from build123d import *

# Parameters (mm, degrees)
BOSS_EXTRUDE1_DEPTH = 60
CUT_EXTRUDE1_DEPTH  = 41
SKETCH3_W           = 20
SKETCH3_H           = 20
CUT_EXTRUDE2_DEPTH  = 10
CHAMFER1_SIZE       = 20
SKETCH4_W           = 10
SKETCH4_H           = 20
CUT_EXTRUDE3_DEPTH  = 30
SKETCH5_W           = 10
SKETCH5_H           = 20
CUT_EXTRUDE4_DEPTH  = 30


with BuildPart() as part:
    # Sketch1 → Boss-Extrude1 (new body)
    with BuildSketch(Plane(origin=(0, 0, 0), x_dir=(1, 0, 0), z_dir=(0, 1, 0))):
        Polygon((0, 0), (60, 0), (60, -40), (30, -40), (30, -20), (0, -20), align=None)
    extrude(amount=BOSS_EXTRUDE1_DEPTH)

    # Sketch2 → Cut-Extrude1 (cut, through all)
    with BuildSketch(Plane.XY.offset(40)):
        Polygon((50, 60), (50, 50), (30, 50), (30, 40), (20, 40), (20, 30), (10, 30), (0, 10), (0, 60), align=None)
    extrude(amount=-CUT_EXTRUDE1_DEPTH, mode=Mode.SUBTRACT)

    # Sketch3 → Cut-Extrude2 (cut)
    with BuildSketch(Plane.XY.offset(20)):
        with Locations((10, 20)):
            Rectangle(SKETCH3_W, SKETCH3_H)
    extrude(amount=-CUT_EXTRUDE2_DEPTH, mode=Mode.SUBTRACT)

    # Chamfer1
    chamfer1_edges = [part.edges().sort_by_distance(p)[0] for p in [
        (55, 60, 40),
    ]]
    chamfer(chamfer1_edges, length=CHAMFER1_SIZE)

    # Sketch4 → Cut-Extrude3 (cut)
    with BuildSketch(Plane(origin=(0, 50, 0), x_dir=(1, 0, 0), z_dir=(0, 1, 0))):
        with Locations((35, -30)):
            Rectangle(SKETCH4_W, SKETCH4_H)
    extrude(amount=-CUT_EXTRUDE3_DEPTH, mode=Mode.SUBTRACT)

    # Sketch5 → Cut-Extrude4 (cut)
    with BuildSketch(Plane.ZY.offset(-30)):
        with Locations((35, 20)):
            Rectangle(SKETCH5_W, SKETCH5_H)
    extrude(amount=-CUT_EXTRUDE4_DEPTH, mode=Mode.SUBTRACT)


solid = part.part
Source: CAD feature listing. Evaluate the final solid. Frame: model axes, mm. A direction names the side the tool comes from. Give positions to 0.01 mm unless a question says otherwise; leave off trailing zeros. Write each loop counter-clockwise with the first axis right and the second up, starting at its lowest first coordinate (ties: lowest second). Pieces come first, ordered by that corner, then holes. Notation, with made-up numbers: M 68,53.5 L 90,53.5 A10 cw 90,62.5 Z; hole C -34.5,35 d8. An arc over 180 degrees is marked long. Return JSON: item names as keys, results as strings. Group by question number.
1) Cut plane A-A, the plane z = 29. Output: boundary loops of the cut face in (x, y), then the cut area to 3 significant figures.
2) Cut plane C-C, the plane x = 44. Output: boundary loops of the cut face in (y, z), then the cut area to 3 significant figures.
3) Cut plane D-D, the plane z = 36.5. Output: boundary loops of the cut face in (x, y).
4) Cut plane B-B, the plane y = 13.5. Output: boundary loops of the cut face in (x, z), then the cut area to 3 significant figures.
5) Set-up query: faces 4 (the face through (12, 20, 10)), 5 (the face through (50, 55, 12)), 6 (the face through (48, 20, 30)), 7 (the face through (52, 48, 32)). Return all of +Z, -Z, +X, -X, +Y, -Y with unobstructed straight access to the full face (end or side cutting, diameter ignored); none if empty.
6) Ray query, L1, parallel to X at y = 34.5, z = 28; L2, parallel to X at y = 38.5, z = 6; L3, parallel to Y at x = 20.5, z = 15. Return the intervals inside material, ascending.
7) First-contact query: pin 1 Ø1.5 at (y, z) = (52.5, 22.5) entering from -X; pin 2 Ø22 at (y, z) = (39, 30.5) entering from -X; pin 3 Ø6 at (y, z) = (24.5, 8.5) entering from -X. Flat tips, straight axial feed; report the tip coordinate or a pass-through.
8) Draft query along Y for faces 1 (the face through (5, 20, 5)), 2 (the face through (30, 8, 28)), 3 (the face through (45, 10, 35)). Return one class per face: released by +Y, released by -Y, zero draft, split by the parting line, or undercut.
Data:
{
 "1": {"outline": "M 30,0 L 60,0 L 60,51 L 50,51 L 50,50 L 40,50 L 40,20 L 30,20 Z", "area": "1,210 mm²"},
 "2": {"outline": "M 0,0 L 50,0 L 50,30 L 40,40 L 30,40 L 30,30 L 10,30 L 10,40 L 0,40 Z", "area": "1,750 mm²"},
 "3": {"outline": "M 30,0 L 60,0 L 60,10 L 30,10 Z; M 40,30 L 60,30 L 60,43.5 L 40,43.5 Z"},
 "4": {"outline": "M 1.75,0 L 60,0 L 60,30 L 30,30 L 30,20 L 20,20 L 20,10 L 1.75,10 Z", "area": "1,280 mm²"},
 "5": {"face 4": "+Z, -X, +Y", "face 5": "+Z, -Z, -X, +Y", "face 6": "+Z, +X, -X", "face 7": "+Z, +X, -X, +Y"},
 "6": {"L1": "x = 40 to 60", "L2": "x = 20 to 60", "L3": "y = 0 to 40"},
 "7": {"pin 1": "stops at x = 50", "pin 2": "stops at x = 20", "pin 3": "stops at x = 5.75"},
 "8": {"face 1": "released by +Y", "face 2": "zero draft", "face 3": "undercut"}
}
